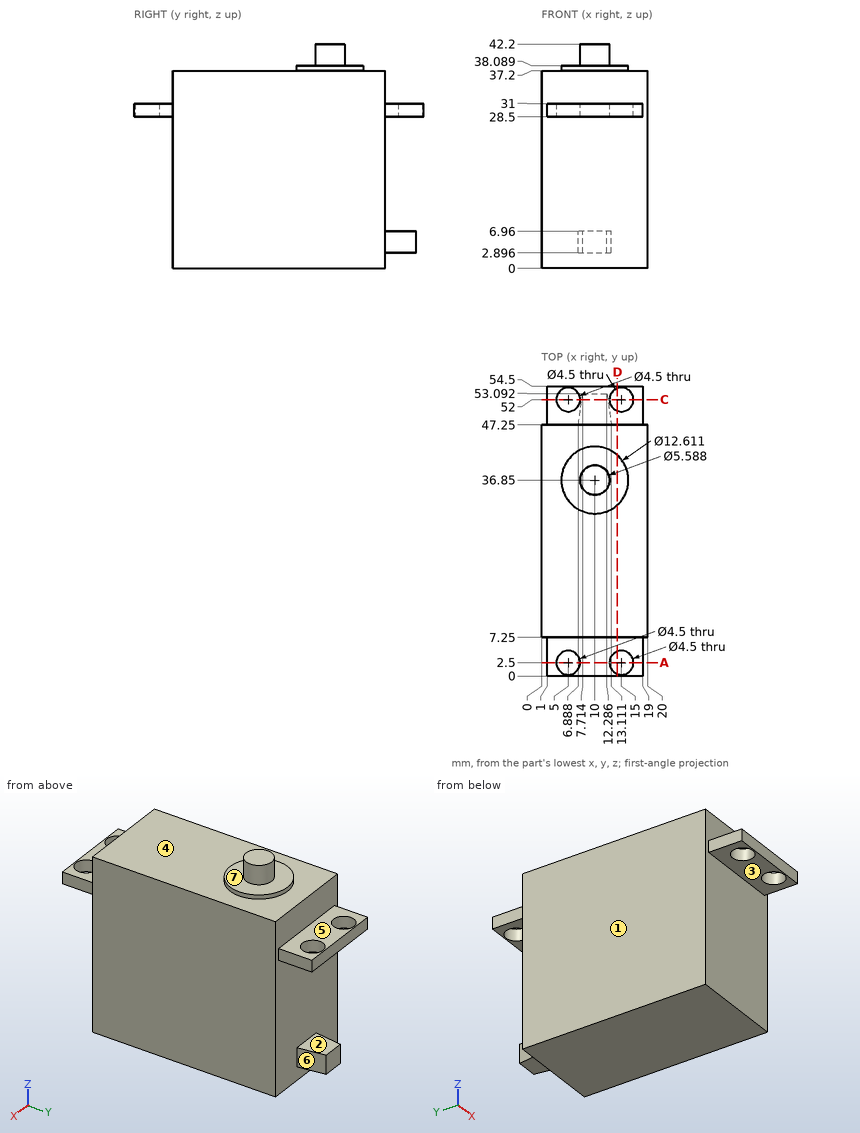
Job drawing, mm, ordinate dimensions from the low corner. One solid piece. A direction names the side the tool comes from. Round coordinates to 2 decimals unless told otherwise and drop trailing zeros. Loops run counter-clockwise (first coordinate to the right, second up) from the corner with the lowest first, then second, coordinate; pieces in that order, holes last. Notation, with made-up numbers: (-20, 79.25) -> (10, 79.25) arc R25 cw to (10, 118.25) -> close; hole circle Ø6 at (42.5, 75). An arc over 180 degrees is marked (long way). One line per item, written item: value. Start each with the question number.
Q1. Cut at C-C on y = 52. Count the separate pieces of the cut face and the enclosed holes in it.
Q2. Two-plate mould, pull along Z, no slides. Class the marked faces 1, 2, 3 and 4: released by +Z, released by -Z, zero draft, split by the parting line, or undercut.
Q3. Cut at D-D on x = 14.25. List the corners of the cut face in (y, z).
Q4. Cut at A-A on y = 2.5. List the corners of the cut face in (x, z), plus the area to 3 significant figures.
Q5. Probe line 1 along Y through (x, z) = (5, 30.55); line 2 along X through (y, z) = (2, 30) (1 decimal); line 3 along Y through (x, z) = (6.75, 16). List the from-to ranges inside material, lowest first.
Q6. Drop flat-ended pins along their axis: pin 1 Ø3.5 at (x, z) = (9.5, 4.5) entering from +Y; pin 2 Ø5 at (x, y) = (8.5, 44) entering from +Z; pin 3 Ø10 at (x, z) = (10, 20.5) entering from +Y. Give the stop position or say it passes through.
Q7. 3-axis set-ups, long thin cutter, end or side, ignore diameter. For the marked faces 5, 6 and 7: which of +Z, -Z, +X, -X, +Y, -Y reach the whole face in a straight line?
Computed:
1. separate pieces: 4
1. enclosed holes: 0
2. face 1: zero draft
2. face 2: undercut
2. face 3: released by -Z
2. face 4: released by +Z
3. outline: (0, 28.5) -> (0.38, 28.5) -> (0.38, 31) -> (0, 31) -> close; (4.62, 28.5) -> (7.25, 28.5) -> (7.25, 0) -> (47.25, 0) -> (47.25, 28.5) -> (49.88, 28.5) -> (49.88, 31) -> (47.25, 31) -> (47.25, 37.2) -> (41.51, 37.2) -> (41.51, 38.09) -> (32.19, 38.09) -> (32.19, 37.2) -> (7.25, 37.2) -> (7.25, 31) -> (4.62, 31) -> close; (54.12, 28.5) -> (54.5, 28.5) -> (54.5, 31) -> (54.12, 31) -> close
4. outline: (1, 28.5) -> (2.75, 28.5) -> (2.75, 31) -> (1, 31) -> close; (7.25, 28.5) -> (12.75, 28.5) -> (12.75, 31) -> (7.25, 31) -> close; (17.25, 28.5) -> (19, 28.5) -> (19, 31) -> (17.25, 31) -> close
4. area: 22.5 mm²
5. line 1: 0 to 0.25, 4.75 to 49.75, 54.25 to 54.5
5. line 2: 1 to 2.8, 7.2 to 12.8, 17.2 to 19
5. line 3: 7.25 to 47.25
6. pin 1: y = 53.09
6. pin 2: z = 38.09
6. pin 3: y = 47.25
7. face 5: +Z, +X, -X, +Y
7. face 6: -Z, +X, +Y
7. face 7: +Z
